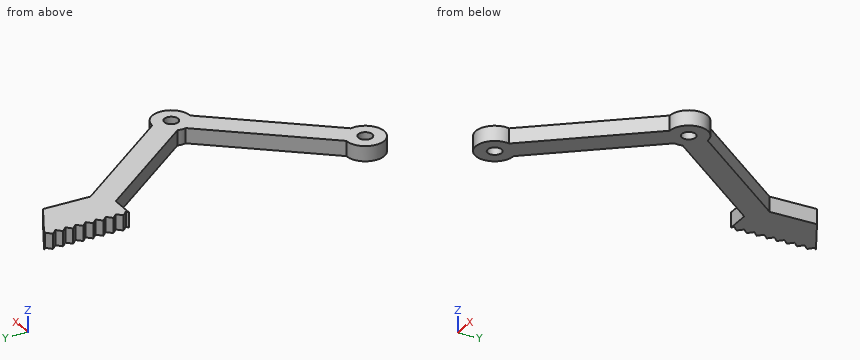
from build123d import *

# Parameters (mm, degrees)
BOSS_EXTRUDE1_DEPTH = 3.18
SKETCH2_R           = 1.47
CUT_EXTRUDE1_DEPTH  = 76.404806599
SKETCH3_R           = 1.47
CUT_EXTRUDE2_DEPTH  = 76.404806599


with BuildPart() as part:
    # Sketch1 → Boss-Extrude1 (new body)
    with BuildSketch(Plane.XY):
        with BuildLine():
            Line((0, 4), (18.75, 27.418742494))
            ThreePointArc((18.75, 27.418742494), (18.653123767, 28.293364452), (18.749834676, 29.168004707))
            Line((18.749834676, 29.168004707), (-0.00459162, 52.583202641))
            Line((-0.00459162, 52.583202641), (-5.00459162, 52.583202641))
            Line((-5.00459162, 52.583202641), (-4.474261534, 52.960989463))
            Line((-4.474261534, 52.960989463), (-5.534921706, 54.021649635))
            Line((-5.534921706, 54.021649635), (-4.474261534, 55.082309806))
            Line((-4.474261534, 55.082309806), (-5.534921706, 56.142969978))
            Line((-5.534921706, 56.142969978), (-4.474261534, 57.20363015))
            Line((-4.474261534, 57.20363015), (-5.534921706, 58.264290322))
            Line((-5.534921706, 58.264290322), (-4.474261534, 59.324950494))
            Line((-4.474261534, 59.324950494), (-5.534921706, 60.385610665))
            Line((-5.534921706, 60.385610665), (-4.474261534, 61.446270837))
            Line((-4.474261534, 61.446270837), (-5.534921706, 62.506931009))
            Line((-5.534921706, 62.506931009), (-4.474261534, 63.567591181))
            Line((-4.474261534, 63.567591181), (-5.534921705, 64.628251353))
            Line((-5.534921705, 64.628251353), (-4.474261534, 65.688911524))
            Line((-4.474261534, 65.688911524), (-5.534921705, 66.749571696))
            Line((-5.534921705, 66.749571696), (-4.474261534, 67.810231868))
            Line((-4.474261534, 67.810231868), (-5.534921705, 68.87089204))
            Line((-5.534921705, 68.87089204), (-4.474261534, 69.931552211))
            Line((-4.474261534, 69.931552211), (-5.00459162, 70.465477027))
            Line((-5.00459162, 70.465477027), (3.831950272, 65.784074737))
            Line((3.831950272, 65.784074737), (3.831950272, 55.784074737))
            Line((3.831950272, 55.784074737), (3.897941369, 55.708940357))
            Line((3.897941369, 55.708940357), (22.652367666, 32.293742423))
            ThreePointArc((22.652367666, 32.293742423), (26.653123731, 28.294120536), (22.653123749, 24.293742494))
            Line((22.653123749, 24.293742494), (3.903123749, 0.875))
            ThreePointArc((3.903123749, 0.875), (-2.5, -3.122498999), (0, 4))
        make_face()
    extrude(amount=BOSS_EXTRUDE1_DEPTH)

    # Sketch2 → Cut-Extrude1 (cut, through all)
    with BuildSketch(Plane(origin=(0, 0, 0), x_dir=(-1, 0, 0), z_dir=(0, 0, -1))):
        with Locations((-22.653123749, 28.293742494)):
            Circle(SKETCH2_R)
    extrude(amount=-CUT_EXTRUDE1_DEPTH, mode=Mode.SUBTRACT)

    # Sketch3 → Cut-Extrude2 (cut, through all)
    with BuildSketch(Plane(origin=(0, 0, 0), x_dir=(-1, 0, 0), z_dir=(0, 0, -1))):
        Circle(SKETCH3_R)
    extrude(amount=-CUT_EXTRUDE2_DEPTH, mode=Mode.SUBTRACT)


solid = part.part
The model under review builds one solid part; all positions refer to its coordinate system, in mm. Coordinates: 2 decimals unless noted, no trailing zeros. Loops run counter-clockwise (first coordinate to the right, second up) from the corner with the lowest first, then second, coordinate; pieces in that order, holes last.
(1) Consider section D-D, the plane y = 31.5. Give the boundary of the cut face in (x, z), plus the area to 3 significant figures.
Determined:
outline: (16.88, 0) - (25.04, 0) - (25.04, 3.18) - (16.88, 3.18) - close
area: 26.0 mm2
(2) Wall thickness on L1, parallel to Y at x = 0, z = 2.35; L2, parallel to Y at x = 5, z = 0.95 (3 decimals); L3, parallel to Y at x = 18, z = 1.2: over which ranges is each line inside the solid? List them lowest first.
Determined:
L1: y = -4 to -1.47, 1.47 to 4, 52.58 to 67.81
L2: y = 2.245 to 10.245, 46.335 to 54.333
L3: y = 18.48 to 26.48, 30.1 to 38.1
(3) Consider section C-C, the plane y = 22. Give the boundary of the cut face in (x, z).
Determined:
outline: (14.41, 0) - (20.82, 0) - (20.82, 3.18) - (14.41, 3.18) - close
(4) Consider section A-A, the plane y = 0. Give the boundary of the cut face in (x, z).
Determined:
outline: (-4, 0) - (-1.47, 0) - (-1.47, 3.18) - (-4, 3.18) - close; (1.47, 0) - (4, 0) - (4, 3.18) - (1.47, 3.18) - close
(5) Consider section B-B, the plane z = 0.85. Give the number of separate pieces and of enclosed holes in the cut face, plus the area to 3 significant figures.
Determined:
separate pieces: 1
enclosed holes: 2
area: 509 mm2
